from build123d import *

# Parameters (mm, degrees)
F0_W     = 1600
F0_H     = 200
F1_DEPTH = 400
F2_T     = -1
F5_D     = 40
F8_D     = 30


# Not quite as in the source:
# - the program builds the solid bodies; features that only make, move or delete a surface that nothing else refers to are left out


with BuildPart() as f1:
    # F0 (on Top) → F1 (new body)
    with BuildSketch(Plane.XY):
        Rectangle(F0_W, F0_H)
    extrude(amount=F1_DEPTH)

    # F2
    f2_openings = [f1.faces().sort_by_distance(p)[0] for p in [
        (0, 0, 400),
    ]]
    offset(amount=F2_T, openings=f2_openings)

    # F5 (through all)
    with Locations(Plane.XY.offset(1)):
        with Locations((777, 77), (777, -77), (-777, 77), (-777, -77)):
            Hole(F5_D / 2)

    # F8 (through all)
    with Locations(Plane(origin=(-800, 0, 0), x_dir=(0, -1, 0), z_dir=(-1, 0, 0))):
        with Locations((0, 50)):
            Hole(F8_D / 2)


solid = f1.part
Input: part model. Units: mm. Frame: model coordinates. A direction names the side the tool comes from. Coordinates: 2 decimals unless noted, no trailing zeros. Order: outer loops, then holes, each group sorted by start corner. A loop starts at its lowest first (then second) coordinate and runs counter-clockwise, first axis right, second up. Notation, with made-up numbers: M 19,68 L 31,68 A17 ccw 31,72 Z; hole C -8.75,-22 d10. An arc over 180 degrees is marked long. Write item = value, one per line. Start each with the question number.
(1) Line query: line 1 along Y through (x, z) = (-777, 0.6); line 2 along X through (y, z) = (-14.5, 340); line 3 along Y through (x, z) = (-618.5, 349). Output: solid intervals per line, ascending. Write a range as [from, to].
(2) Pull-direction query (X, two-part tool) for faces 1 (the flat face through (-11, 100, 197)), 2 (the flat face through (800, -1, 197)), 3 (the flat face through (-799, -1, 198)); classes: released by +X, released by -X, zero draft, split by the parting line, or undercut.
(3) Section D-D on x = 690. Output: boundary loops of the cut face in (y, z), and give its area (3 significant figures).
(4) Section B-B on x = -777. Output: boundary loops of the cut face in (y, z).
(5) First-contact query: P1, Ø10, axis at x = -399, y = 58, coming from the +Z side; P2, Ø18, axis at y = 0, z = 50, coming from the -X side (3 decimals). Flat tips, straight axial feed; report the tip coordinate or a pass-through.
(6) Section A-A on y = 0. Output: boundary loops of the cut face in (x, z).
(7) Reachability of faces 4 (the cylindrical face through (-761.13, 64.83, 0.49)), 5 (the flat face through (-11, 1, 1)) from +Z, -Z, +X, -X, +Y, -Y: full face, straight path, thin tool, end or side. Return the list, or none.
(8) Section C-C on z = 50. Output: boundary loops of the cut face in (x, y), and give its area (3 significant figures).
Result set:
q1.line_1 = [-100, -97], [-57, 57], [97, 100]
q1.line_2 = [-800, -799], [799, 800]
q1.line_3 = [-100, -99], [99, 100]
q2.face_1 = zero draft
q2.face_2 = released by +X
q2.face_3 = undercut
q3.outline = M -100,0 L 100,0 L 100,400 L 99,400 L 99,1 L -99,1 L -99,400 L -100,400 Z
q3.area = 998 mm²
q4.outline = M -100,0 L -97,0 L -97,1 L -99,1 L -99,400 L -100,400 Z; M -57,0 L 57,0 L 57,1 L -57,1 Z; M 97,0 L 100,0 L 100,400 L 99,400 L 99,1 L 97,1 Z
q5.P1 = 1
q5.P2 = through
q6.outline = M -800,0 L 800,0 L 800,35 L 799,35 L 799,1 L -799,1 L -799,35 L -800,35 Z; M -800,65 L -799,65 L -799,400 L -800,400 Z; M 799,65 L 800,65 L 800,400 L 799,400 Z
q7.face_4 = +Z, -Z
q7.face_5 = +Z
q8.outline = M -800,-100 L 800,-100 L 800,-15 L 799,-15 L 799,-99 L -799,-99 L -799,-15 L -800,-15 Z; M -800,15 L -799,15 L -799,99 L 799,99 L 799,15 L 800,15 L 800,100 L -800,100 Z
q8.area = 3,540 mm²
